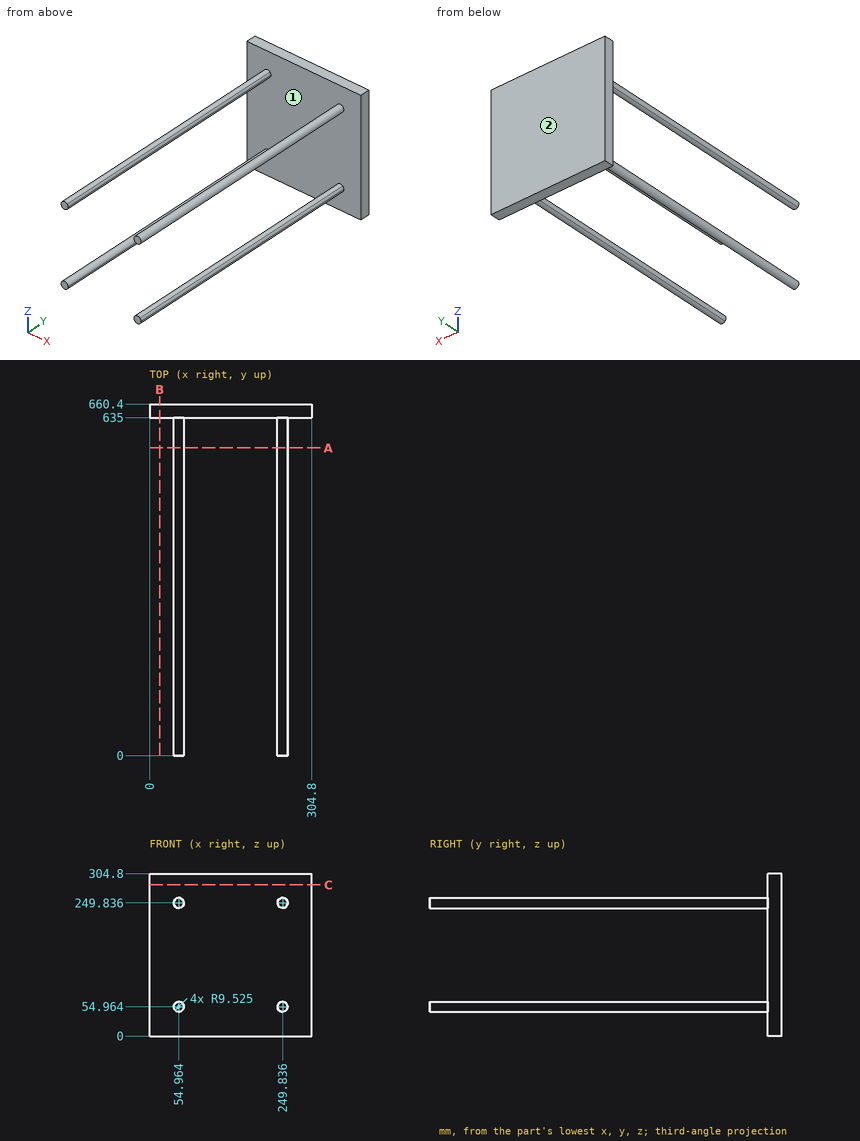
Print and shaded views of the part. All mm, measured from the part's lowest x, y and z. A direction names the side the tool comes from. Round coordinates to 2 decimals unless told otherwise and drop trailing zeros. Order: outer loops, then holes, each group sorted by start corner. A loop starts at its lowest first (then second) coordinate and runs counter-clockwise, first axis right, second up.
Q1. Slice it at B-B (x = 19). Write the cut outline in (y, z).
Q2. Slice it at C-C (z = 284). Write the cut outline in (x, y).
Q3. Slice it at A-A (y = 578). State how many separate pieces and enclosed holes the cut face has, and give its area (3 significant figures).
Q4. Drop flat-ended pins along their axis: pin 1 (10 mm diameter, centred on x = 251, z = 77.5, fed in from -Y); pin 2 (3 mm diameter, centred on y = 424, z = 61.5, fed in from -X). Give the stop position or say it passes through.
Q5. Wall check: L1, parallel to Y at x = 69.5, z = 31; L2, parallel to Z at x = 53, y = 373.5 (1 decimal). Give the ranges that are in metal, low to high.
Q6. Which spindle directions (+Z, -Z, +X, -X, +Y, -Y) get a long thin tool onto all of the face, cutting with end or side? Do the marked faces 1 and 2. Say none if no direction does.
Results below:
1. outline: (635, 0) - (660.4, 0) - (660.4, 304.8) - (635, 304.8) - close
2. outline: (0, 635) - (304.8, 635) - (304.8, 660.4) - (0, 660.4) - close
3. separate pieces: 4
3. enclosed holes: 0
3. area: 1,140 mm2
4. pin 1: stops at y = 635
4. pin 2: stops at x = 46.88
5. L1: y = 635 to 660.4
5. L2: z = 45.6 to 64.3, 240.5 to 259.2
6. face 1: -Y
6. face 2: +Z, -Z, +X, -X, +Y
